```python
from build123d import *

# Parameters (mm, degrees)
F0_R     = 6.35
F1_DEPTH = 25.4


with BuildPart() as f1:
    # F0 (on Front) → F1 (new body)
    with BuildSketch(Plane.XZ):
        Polygon((29.156278, 14.92035), (-30.525118, 14.92035), (-49.141338, 0), (-49.141338, -4.790938), (-45.308587, -16.28919), (-30.525118, -23.95469), (37.643085, -23.95469), (47.224959, -16.28919), (44.487282, 0), (37.643085, 8.623689), align=None)
        with Locations((-18.753101, -13.551511)):
            Circle(F0_R, mode=Mode.SUBTRACT)
        with Locations((17.384261, -13.825279)):
            Circle(F0_R, mode=Mode.SUBTRACT)
    extrude(amount=F1_DEPTH)


solid = f1.part
```
Source: CAD feature listing. Evaluate the final solid. Frame: model axes, mm. Give positions to 0.01 mm unless a question says otherwise; leave off trailing zeros. Write each loop counter-clockwise with the first axis right and the second up, starting at its lowest first coordinate (ties: lowest second). Pieces come first, ordered by that corner, then holes. Notation, with made-up numbers: (41.25, 13.25) - (69.25, 13.25) arc R13 ccw to (69.25, 24.25) - close; hole circle Ø2 at (35.5, 84). An arc over 180 degrees is marked (long way). One line per item, written item: value. Start each with the question number.
Q1. First-contact query: pin 1 Ø10 at (y, z) = (-8, 0) entering from +X; pin 2 Ø1.5 at (y, z) = (-16.5, 0.5) entering from +X; pin 3 Ø11.5 at (x, z) = (-18.75, -13.55) entering from -Y; pin 4 Ø5 at (y, z) = (-18.5, -12) entering from +X. Flat tips, straight axial feed; report the tip coordinate or a pass-through.
Q2. Section query B-B, the plane y = -23. Return the cut outline in (x, z), then the cut area to 3 significant figures.
Q3. Section query D-D, the plane x = -17.5. Return the cut outline in (y, z), then the cut area to 3 significant figures.
Q4. Section query C-C, the plane z = -15. Return the cut outline in (x, y).
Q5. Draft query along X for faces 1 (the face through (-2, -25.4, -4)), 2 (the face through (-23.79, -12.52, -17.42)), 3 (the face through (-49.141, -13, -2)). Return one class per face: +X half, -X half, draft (parallel to the pull), parting line (faces both ways), or undercut.
Q6. Material intervals for probe 1 along X at (y, z) = (-13.5, -13.5); probe 2 along X at (y, z) = (-21.5, -14.5); probe 3 along X at (y, z) = (-18, 0), sorted ascending. Write a range as from..to.
Q7. Section query A-A, the plane x = 17. Return the cut outline in (y, z), then the cut area to 3 significant figures.
Answer:
1. pin 1: stops at x = 45.33
1. pin 2: stops at x = 44.53
1. pin 3: passes through
1. pin 4: stops at x = 46.92
2. outline: (-49.14, -4.79) - (-45.31, -16.29) - (-30.53, -23.95) - (37.64, -23.95) - (47.22, -16.29) - (44.49, 0) - (37.64, 8.62) - (29.16, 14.92) - (-30.53, 14.92) - (-49.14, 0) - close; hole circle Ø12.7 at (-18.75, -13.55); hole circle Ø12.7 at (17.38, -13.83)
2. area: 3,050 mm2
3. outline: (-25.4, -23.95) - (0, -23.95) - (0, -19.78) - (-25.4, -19.78) - close; (-25.4, -7.33) - (0, -7.33) - (0, 14.92) - (-25.4, 14.92) - close
3. area: 671 mm2
4. outline: (-45.74, -25.4) - (-24.94, -25.4) - (-24.94, 0) - (-45.74, 0) - close; (-12.57, -25.4) - (11.14, -25.4) - (11.14, 0) - (-12.57, 0) - close; (23.62, -25.4) - (47.01, -25.4) - (47.01, 0) - (23.62, 0) - close
5. face 1: draft
5. face 2: undercut
5. face 3: -X half
6. probe 1: x = -46.24..-25.1, -12.4..11.04, 23.73..46.76
6. probe 2: x = -45.9..-25.03, -12.47..11.07, 23.7..46.92
6. probe 3: x = -49.14..44.49
7. outline: (-25.4, -23.95) - (0, -23.95) - (0, -20.16) - (-25.4, -20.16) - close; (-25.4, -7.49) - (0, -7.49) - (0, 14.92) - (-25.4, 14.92) - close
7. area: 665 mm2
